Read the model definition and answer for the solid it produces. Units are mm, in the model's axes. A direction names the side the tool comes from. Coordinates: 2 decimals unless noted, no trailing zeros. Loops run counter-clockwise (first coordinate to the right, second up) from the corner with the lowest first, then second, coordinate; pieces in that order, holes last.
Q1. Section B-B (x = 0) is taken. Give the vertices of the cut face in (y, z).
Q2. Which of the six approach directions +Z, -Z, +X, -X, +Y, -Y give full straight-line access (tool end or side, diameter ignored) to faces 5 (the face through (0, -28, 2)), 6 (the face through (2.3, 0, 2)), 7 (the face through (-0.9, -4.05, 4.49))?
Q3. Straight lines are drawn through the part: line 1 (Y direction, x = 10, z = -28); line 2 (Z direction, x = 3, y = 1); line 3 (X direction, y = -14, z = -1.5). For each, find the intervals that lie inside material, in ascending order.
Q4. The mould has two halves that part along Y. Classify faces 1 (the face through (3, -25, 3.5)), 2 (the face through (-15, -17, -26)), 3 (the face through (0.2, -8.4, -42.2)), 4 (the face through (0, -12, 0)): pulls with the +Y half, pulls with the -Y half, needs draft (parallel to the pull), parting line crosses it, or undercut.
Q5. Section A-A (y = 0) is taken. Give the vertices of the cut face in (x, z).
Q6. Section D-D (y = -6) is taken. Give the vertices of the cut face in (x, z), then the cut area to 3 significant figures.
Q7. Flat-ended cylindrical pins translate along their axes: P1, Ø5, axis at x = -6, z = -35, coming from the -Y side; P2, Ø6.5, axis at x = 0.5, y = -1.5, coming from the -Z side; P3, Ø3, axis at x = 0, y = -7.5, coming from the -Z side. Find the tip coordinate at first contact, or state that the pin passes through.
Q8. Section C-C (z = -21) is taken. Give the vertices of the cut face in (x, y), then the cut area to 3 significant figures.
from build123d import *

# Parameters (mm, degrees)
EXTRUDE_1_DEPTH   = 3.5
EXTRUDE_1_2_DEPTH = 3.5
SKETCH_2_R        = 4.15
EXTRUDE_2_DEPTH   = 2
SKETCH_3_W        = 10
SKETCH_3_H        = 38
EXTRUDE_3_DEPTH   = 4.5
SKETCH_5_W        = 30
SKETCH_5_H        = 6
EXTRUDE_4_DEPTH   = 25
EXTRUDE_5_DEPTH   = 6
SKETCH_10_W       = 30
SKETCH_10_H       = 6
SKETCH_11_W       = 30
SKETCH_11_H       = 3
REVOLVE_1_ANGLE   = 180
FILLET_1_R        = 3


with BuildPart() as part:
    # Sketch 1 → Extrude 1 (new body)
    with BuildSketch(Plane.XY):
        with BuildLine():
            Line((-2.3, 1.926136028), (-2.3, -1.926136028))
            ThreePointArc((-2.3, -1.926136028), (0, -3), (2.3, -1.926136028))
            Line((2.3, -1.926136028), (2.3, 1.926136028))
            ThreePointArc((2.3, 1.926136028), (0, 3), (-2.3, 1.926136028))
        make_face()
    extrude(amount=EXTRUDE_1_DEPTH)



with BuildPart() as body_2:
    # Sketch 1 → Extrude 1 2 (new body)
    with BuildSketch(Plane.XY):
        with BuildLine():
            Line((-2.3, -23.073863972), (-2.3, -26.926136028))
            ThreePointArc((-2.3, -26.926136028), (0, -28), (2.3, -26.926136028))
            Line((2.3, -26.926136028), (2.3, -23.073863972))
            ThreePointArc((2.3, -23.073863972), (0, -22), (-2.3, -23.073863972))
        make_face()
    extrude(amount=EXTRUDE_1_2_DEPTH)


with BuildPart() as part_1:
    add(part.part)

    add(body_2.part)  # Extrude 2 merges body 2
    # Sketch 2 → Extrude 2 (add)
    with BuildSketch(Plane.XY.offset(3.5)):
        Circle(SKETCH_2_R)
        with Locations((0, -25)):
            Circle(SKETCH_2_R)
    extrude(amount=EXTRUDE_2_DEPTH)

    # Sketch 3 → Extrude 3 (add)
    with BuildSketch(Plane(origin=(0, 0, 0), x_dir=(-1, 0, 0), z_dir=(0, 0, -1))):
        with Locations((0, -12.5)):
            Rectangle(SKETCH_3_W, SKETCH_3_H)
    extrude(amount=EXTRUDE_3_DEPTH)

    # Sketch 5 → Extrude 4 (add)
    with BuildSketch(Plane(origin=(0, 0, -4.5), x_dir=(-1, 0, 0), z_dir=(0, 0, -1))):
        with Locations((0, -18.5)):
            Rectangle(SKETCH_5_W, SKETCH_5_H)
    extrude(amount=EXTRUDE_4_DEPTH)

    # Sketch 8 → Extrude 5 (add)
    with BuildSketch(Plane(origin=(0, -15.5, 0), x_dir=(1, 0, 0), z_dir=(0, 1, 0))):
        Polygon((15, 4.5), (5, 4.5), (5, 0), align=None)
        Polygon((-15, 4.5), (-5, 4.5), (-5, 0), align=None)
    extrude(amount=-EXTRUDE_5_DEPTH)

    # Sweep 1: sweep along a path in Sketch 9
    with BuildLine(Plane(origin=(0, 0, 0), x_dir=(0, 0, -1), z_dir=(1, 0, 0))) as sweep_1_path:
        Line((29.5, -18.5), (34.5, -18.5))
        ThreePointArc((34.5, -18.5), (36, -18.098076211), (37.098076211, -17))
        Line((37.098076211, -17), (40.598076211, -10.937822174))
    # Sketch 10 → Sweep 1 (sweep)
    with BuildSketch(Plane(origin=(0, 0, -29.5), x_dir=(-1, 0, 0), z_dir=(0, 0, -1))):
        with Locations((0, -18.5)):
            Rectangle(SKETCH_10_W, SKETCH_10_H)
    sweep(path=sweep_1_path.line)

    # Sketch 11 → Revolve 1 (revolve)
    with BuildSketch(Plane(origin=(0, 9.376116042, -5.413303121), x_dir=(1, 0, 0), z_dir=(0, 0.866025404, -0.5))):
        with Locations((0, 42.127876431)):
            Rectangle(SKETCH_11_W, SKETCH_11_H)
    revolve(axis=Axis((15, -10.937822174, -40.598076211), (1, 0, 0)), revolution_arc=REVOLVE_1_ANGLE)

    # Fillet 1
    fillet_1_edges = [part_1.edges().sort_by_distance(p)[0] for p in [
        (15, -18.5, -4.5),
        (-15, -18.5, -4.5),
    ]]
    fillet(fillet_1_edges, radius=FILLET_1_R)


solid = part_1.part
Numbers:
1. outline: (-31.5, -4.5) - (-21.5, -4.5) - (-21.5, -34.5) arc R6 ccw to (-18.5, -39.7) - (-12.44, -43.2) arc R3 ccw to (-9.44, -38) - (-15.5, -34.5) - (-15.5, -4.5) - (6.5, -4.5) - (6.5, 0) - (3, 0) - (3, 3.5) - (4.15, 3.5) - (4.15, 5.5) - (-4.15, 5.5) - (-4.15, 3.5) - (-3, 3.5) - (-3, 0) - (-22, 0) - (-22, 3.5) - (-20.85, 3.5) - (-20.85, 5.5) - (-29.15, 5.5) - (-29.15, 3.5) - (-28, 3.5) - (-28, 0) - (-31.5, 0) - close
2. face 5: -Y
2. face 6: +X, +Y, -Y
2. face 7: +Z
3. line 1: y = -21.5 to -15.5
3. line 2: z = -4.5 to 0, 3.5 to 5.5
3. line 3: x = -5 to 5
4. face 1: undercut
4. face 2: needs draft
4. face 3: parting line crosses it
4. face 4: undercut
5. outline: (-5, -4.5) - (5, -4.5) - (5, 0) - (2.3, 0) - (2.3, 3.5) - (4.15, 3.5) - (4.15, 5.5) - (-4.15, 5.5) - (-4.15, 3.5) - (-2.3, 3.5) - (-2.3, 0) - (-5, 0) - close
6. outline: (-5, -4.5) - (5, -4.5) - (5, 0) - (-5, 0) - close
6. area: 45.0 mm2
7. P1: stops at y = -21.5
7. P2: stops at z = -4.5
7. P3: stops at z = -42.89
8. outline: (-15, -21.5) - (15, -21.5) - (15, -15.5) - (-15, -15.5) - close
8. area: 180 mm2
